For this review, take the finished solid that the model builds, in its own axes (mm). Round coordinates to 2 decimals unless told otherwise and drop trailing zeros. Order: outer loops, then holes, each group sorted by start corner. A loop starts at its lowest first (then second) coordinate and runs counter-clockwise, first axis right, second up.
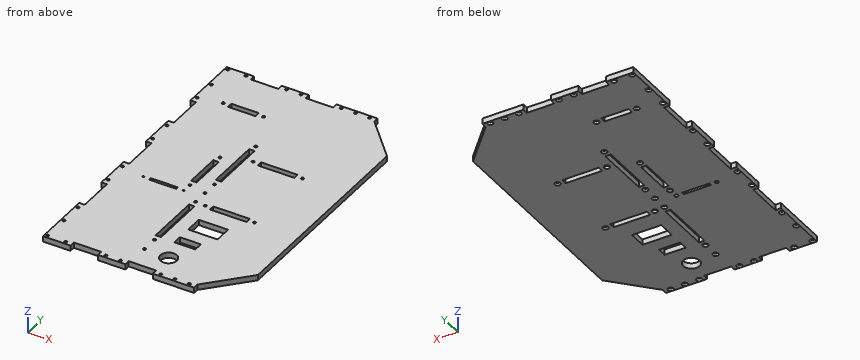
```python
from build123d import *

# Parameters (mm, degrees)
ESQUISSE1_W             = 148
ESQUISSE1_H             = 330
BOSS_EXTRU_1_DEPTH      = 6
ESQUISSE2_W             = 30
ESQUISSE2_H             = 6
ESQUISSE2_W_2           = 6
ESQUISSE2_H_2           = 40
ENL_V_MAT_EXTRU_1_DEPTH = 6
ESQUISSE5_R             = 9
ESQUISSE5_W             = 30
ESQUISSE5_H             = 6
ESQUISSE5_W_2           = 32
ESQUISSE5_H_2           = 19
ESQUISSE5_W_3           = 23
ESQUISSE5_H_3           = 10
ESQUISSE5_H_4           = 3
ENL_V_MAT_EXTRU_3_DEPTH = 6
ESQUISSE6_W             = 6
ESQUISSE6_H             = 60
ENL_V_MAT_EXTRU_4_DEPTH = 10
ESQUISSE8_W             = 6
ESQUISSE8_H             = 330
BOSS_EXTRU_2_DEPTH      = 57
ENL_V_MAT_EXTRU_5_DEPTH = 389.536999525
ESQUISSE10_W            = 6
ESQUISSE10_H            = 40
ESQUISSE10_W_2          = 40
ESQUISSE10_H_2          = 6
ENL_V_MAT_EXTRU_6_DEPTH = 389.536999525
ESQUISSE11_R            = 1.5
ESQUISSE11_R_2          = 1.005
ENL_V_MAT_EXTRU_7_DEPTH = 389.536999525
ESQUISSE12_R            = 2.995
ESQUISSE12_R_2          = 3
ESQUISSE12_R_3          = 2
ENL_V_MAT_EXTRU_8_DEPTH = 3


with BuildPart() as part:
    # Esquisse1 → Boss.-Extru.1 (new body)
    with BuildSketch(Plane.XY):
        with Locations((74, 165)):
            Rectangle(ESQUISSE1_W, ESQUISSE1_H)
    extrude(amount=BOSS_EXTRU_1_DEPTH)

    # Esquisse2 → Enlèv. mat.-Extru.1 (cut)
    with BuildSketch(Plane.XY.offset(6)):
        with Locations((45, 3)):
            Rectangle(ESQUISSE2_W, ESQUISSE2_H)
        with Locations((105, 3)):
            Rectangle(ESQUISSE2_W, ESQUISSE2_H)
        with Locations((45, 327)):
            Rectangle(ESQUISSE2_W, ESQUISSE2_H)
        with Locations((105, 327)):
            Rectangle(ESQUISSE2_W, ESQUISSE2_H)
        with Locations((3, 245)):
            Rectangle(ESQUISSE2_W_2, ESQUISSE2_H_2)
        with Locations((3, 165)):
            Rectangle(ESQUISSE2_W_2, ESQUISSE2_H_2)
        with Locations((3, 85)):
            Rectangle(ESQUISSE2_W_2, ESQUISSE2_H_2)
    extrude(amount=-ENL_V_MAT_EXTRU_1_DEPTH, mode=Mode.SUBTRACT)

    # Esquisse5 → Enlèv. mat.-Extru.3 (cut)
    with BuildSketch(Plane.XY.offset(6)):
        with Locations((119, 30)):
            Circle(ESQUISSE5_R)
        with Locations((50.5, 277)):
            Rectangle(ESQUISSE5_W, ESQUISSE5_H)
        with Locations((126, 89.5)):
            Rectangle(ESQUISSE5_W_2, ESQUISSE5_H_2)
        with Locations((121.5, 60)):
            Rectangle(ESQUISSE5_W_3, ESQUISSE5_H_3)
        with Locations((50.5, 133.5)):
            Rectangle(ESQUISSE5_W, ESQUISSE5_H_4)
    extrude(amount=-ENL_V_MAT_EXTRU_3_DEPTH, mode=Mode.SUBTRACT)

    # Esquisse6 → Enlèv. mat.-Extru.4 (cut)
    with BuildSketch(Plane.XY.offset(6)):
        with Locations((92, 86)):
            Rectangle(ESQUISSE6_W, ESQUISSE6_H)
        with Locations((92, 194)):
            Rectangle(ESQUISSE6_W, ESQUISSE6_H)
    extrude(amount=-ENL_V_MAT_EXTRU_4_DEPTH, mode=Mode.SUBTRACT)

    # Esquisse8 → Boss.-Extru.2 (add)
    with BuildSketch(Plane(origin=(148, 0, 0), x_dir=(0, 0, -1), z_dir=(1, 0, 0))):
        with Locations((-3, 165)):
            Rectangle(ESQUISSE8_W, ESQUISSE8_H)
    extrude(amount=BOSS_EXTRU_2_DEPTH)

    # Esquisse9 → Enlèv. mat.-Extru.5 (cut, through all)
    with BuildSketch(Plane.XY.offset(6)):
        Polygon((165, 0), (205, 0), (205, 49), (165, 6), align=None)
        Polygon((165, 330), (205, 330), (205, 281), (165, 324), align=None)
    extrude(amount=-ENL_V_MAT_EXTRU_5_DEPTH, mode=Mode.SUBTRACT)

    # Esquisse10 → Enlèv. mat.-Extru.6 (cut, through all)
    with BuildSketch(Plane.XY.offset(6)):
        with Locations((73, 171)):
            Rectangle(ESQUISSE10_W, ESQUISSE10_H)
        with Locations((130, 208)):
            Rectangle(ESQUISSE10_W_2, ESQUISSE10_H_2)
        with Locations((130, 122)):
            Rectangle(ESQUISSE10_W_2, ESQUISSE10_H_2)
    extrude(amount=-ENL_V_MAT_EXTRU_6_DEPTH, mode=Mode.SUBTRACT)

    # Esquisse11 → Enlèv. mat.-Extru.7 (cut, through all)
    with BuildSketch(Plane.XY.offset(6)):
        with Locations((158, 327)):
            Circle(ESQUISSE11_R)
        with Locations((142.5, 327)):
            Circle(ESQUISSE11_R)
        with Locations((127, 327)):
            Circle(ESQUISSE11_R)
        with Locations((67, 327)):
            Circle(ESQUISSE11_R)
        with Locations((83, 327)):
            Circle(ESQUISSE11_R)
        with Locations((3, 327)):
            Circle(ESQUISSE11_R)
        with Locations((23, 327)):
            Circle(ESQUISSE11_R)
        with Locations((3, 297.5)):
            Circle(ESQUISSE11_R)
        with Locations((3, 272)):
            Circle(ESQUISSE11_R)
        with Locations((3, 218)):
            Circle(ESQUISSE11_R)
        with Locations((3, 192)):
            Circle(ESQUISSE11_R)
        with Locations((3, 138)):
            Circle(ESQUISSE11_R)
        with Locations((3, 112)):
            Circle(ESQUISSE11_R)
        with Locations((3, 58)):
            Circle(ESQUISSE11_R)
        with Locations((3, 3)):
            Circle(ESQUISSE11_R)
        with Locations((3, 32.5)):
            Circle(ESQUISSE11_R)
        with Locations((23, 3)):
            Circle(ESQUISSE11_R)
        with Locations((67, 3)):
            Circle(ESQUISSE11_R)
        with Locations((83, 3)):
            Circle(ESQUISSE11_R)
        with Locations((127, 3)):
            Circle(ESQUISSE11_R)
        with Locations((158, 3)):
            Circle(ESQUISSE11_R)
        with Locations((142.5, 3)):
            Circle(ESQUISSE11_R)
        with Locations((92, 231)):
            Circle(ESQUISSE11_R)
        with Locations((92, 157)):
            Circle(ESQUISSE11_R)
        with Locations((92, 123)):
            Circle(ESQUISSE11_R)
        with Locations((92, 49)):
            Circle(ESQUISSE11_R)
        with Locations((92, 140)):
            Circle(ESQUISSE11_R)
        with Locations((73, 144)):
            Circle(ESQUISSE11_R)
        with Locations((73, 198)):
            Circle(ESQUISSE11_R)
        with Locations((28.5, 133.5)):
            Circle(ESQUISSE11_R_2)
        with Locations((72.5, 133.5)):
            Circle(ESQUISSE11_R_2)
        with Locations((72.5, 277)):
            Circle(ESQUISSE11_R)
        with Locations((28.5, 277)):
            Circle(ESQUISSE11_R)
        with Locations((92, 31)):
            Circle(ESQUISSE11_R)
        with Locations((103, 208)):
            Circle(ESQUISSE11_R)
        with Locations((157, 208)):
            Circle(ESQUISSE11_R)
        with Locations((157, 122)):
            Circle(ESQUISSE11_R)
        with Locations((103, 122)):
            Circle(ESQUISSE11_R)
    extrude(amount=-ENL_V_MAT_EXTRU_7_DEPTH, mode=Mode.SUBTRACT)

    # Esquisse12 → Enlèv. mat.-Extru.8 (cut)
    with BuildSketch(Plane(origin=(0, 0, 0), x_dir=(-1, 0, 0), z_dir=(0, 0, -1))):
        with Locations((-158, 327)):
            Circle(ESQUISSE12_R)
        with Locations((-142.5, 327)):
            Circle(ESQUISSE12_R)
        with Locations((-127, 327)):
            Circle(ESQUISSE12_R)
        with Locations((-83, 327)):
            Circle(ESQUISSE12_R)
        with Locations((-67, 327)):
            Circle(ESQUISSE12_R)
        with Locations((-23, 327)):
            Circle(ESQUISSE12_R)
        with Locations((-3, 327)):
            Circle(ESQUISSE12_R)
        with Locations((-3, 297.5)):
            Circle(ESQUISSE12_R)
        with Locations((-3, 272)):
            Circle(ESQUISSE12_R)
        with Locations((-28.5, 277)):
            Circle(ESQUISSE12_R_2)
        with Locations((-72.5, 277)):
            Circle(ESQUISSE12_R_2)
        with Locations((-92, 231)):
            Circle(ESQUISSE12_R_2)
        with Locations((-103, 208)):
            Circle(ESQUISSE12_R_2)
        with Locations((-73, 144)):
            Circle(ESQUISSE12_R_2)
        with Locations((-3, 218)):
            Circle(ESQUISSE12_R)
        with Locations((-3, 192)):
            Circle(ESQUISSE12_R)
        with Locations((-73, 198)):
            Circle(ESQUISSE12_R_2)
        with Locations((-92, 157)):
            Circle(ESQUISSE12_R_2)
        with Locations((-92, 140)):
            Circle(ESQUISSE12_R_2)
        with Locations((-92, 123)):
            Circle(ESQUISSE12_R_2)
        with Locations((-72.5, 133.5)):
            Circle(ESQUISSE12_R_3)
        with Locations((-28.5, 133.5)):
            Circle(ESQUISSE12_R_3)
        with Locations((-3, 112)):
            Circle(ESQUISSE12_R)
        with Locations((-3, 138)):
            Circle(ESQUISSE12_R)
        with Locations((-3, 58)):
            Circle(ESQUISSE12_R)
        with Locations((-3, 32.5)):
            Circle(ESQUISSE12_R)
        with Locations((-3, 3)):
            Circle(ESQUISSE12_R)
        with Locations((-23, 3)):
            Circle(ESQUISSE12_R)
        with Locations((-67, 3)):
            Circle(ESQUISSE12_R)
        with Locations((-83, 3)):
            Circle(ESQUISSE12_R)
        with Locations((-92, 31)):
            Circle(ESQUISSE12_R_2)
        with Locations((-92, 49)):
            Circle(ESQUISSE12_R_2)
        with Locations((-127, 3)):
            Circle(ESQUISSE12_R)
        with Locations((-142.5, 3)):
            Circle(ESQUISSE12_R)
        with Locations((-157, 208)):
            Circle(ESQUISSE12_R_2)
        with Locations((-158, 3)):
            Circle(ESQUISSE12_R)
        with Locations((-157, 122)):
            Circle(ESQUISSE12_R_2)
        with Locations((-103, 122)):
            Circle(ESQUISSE12_R_2)
    extrude(amount=-ENL_V_MAT_EXTRU_8_DEPTH, mode=Mode.SUBTRACT)


solid = part.part
```
Q1. Take a section at A-A, the plane y = 90. State the section outline as (x, z) points.
Q2. Wall thickness on line 1 (Y direction, x = 83, z = 4.2); line 2 (X direction, y = 96, z = 3.05); line 3 (X direction, y = 168.5, z = 3.7): over which ranges is each line inside the solid? List them lowest first.
Q3. Take a section at B-B, the plane z = 4.4. Count the separate pieces of the cut face and the enclosed holes in it, plus the area to 3 significant figures.
Q4. Clearance check with flat-ended pins moving along their axes: pin 1 (1.8 mm diameter, centred on x = 54, z = 1.5, fed in from -Y); pin 2 (3 mm diameter, centred on x = 57, z = 1.5, fed in from +Y); pin 3 (2.5 mm diameter, centred on x = 28.5, y = 133.5, fed in from -Z); pin 4 (2.5 mm diameter, centred on x = 23, y = 327, fed in from -Z). State where each tip first meets the part, or that it passes through.
Q5. Take a section at C-C, the plane x = 177. State the section outline as (y, z) points, plus the area to 3 significant figures.
Working result:
1. outline: (6, 0) - (89, 0) - (89, 6) - (6, 6) - close; (95, 0) - (110, 0) - (110, 6) - (95, 6) - close; (142, 0) - (205, 0) - (205, 6) - (142, 6) - close
2. line 1: y = 0 to 1.5, 4.5 to 325.5, 328.5 to 330
2. line 2: x = 6 to 89, 95 to 110, 142 to 205
2. line 3: x = 6 to 70, 76 to 89, 95 to 205
3. separate pieces: 1
3. enclosed holes: 48
3. area: 60,900 mm2
4. pin 1: stops at y = 6
4. pin 2: stops at y = 324
4. pin 3: stops at z = 3
4. pin 4: passes through
5. outline: (18.9, 0) - (311.1, 0) - (311.1, 6) - (18.9, 6) - close
5. area: 1,750 mm2
